Geometry: see drawing. Coordinates: mm, zero at the bounding-box minimum. A direction names the side the tool comes from. Round coordinates to 2 decimals unless told otherwise and drop trailing zeros. Loops run counter-clockwise (first coordinate to the right, second up) from the corner with the lowest first, then second, coordinate; pieces in that order, holes last. Notation, with made-up numbers: M 34,4 L 65,4 A30 ccw 65,39 Z; hole C 27.5,-32.75 d6. An arc over 180 degrees is marked long. Answer as a JSON object with one key per item and string values.
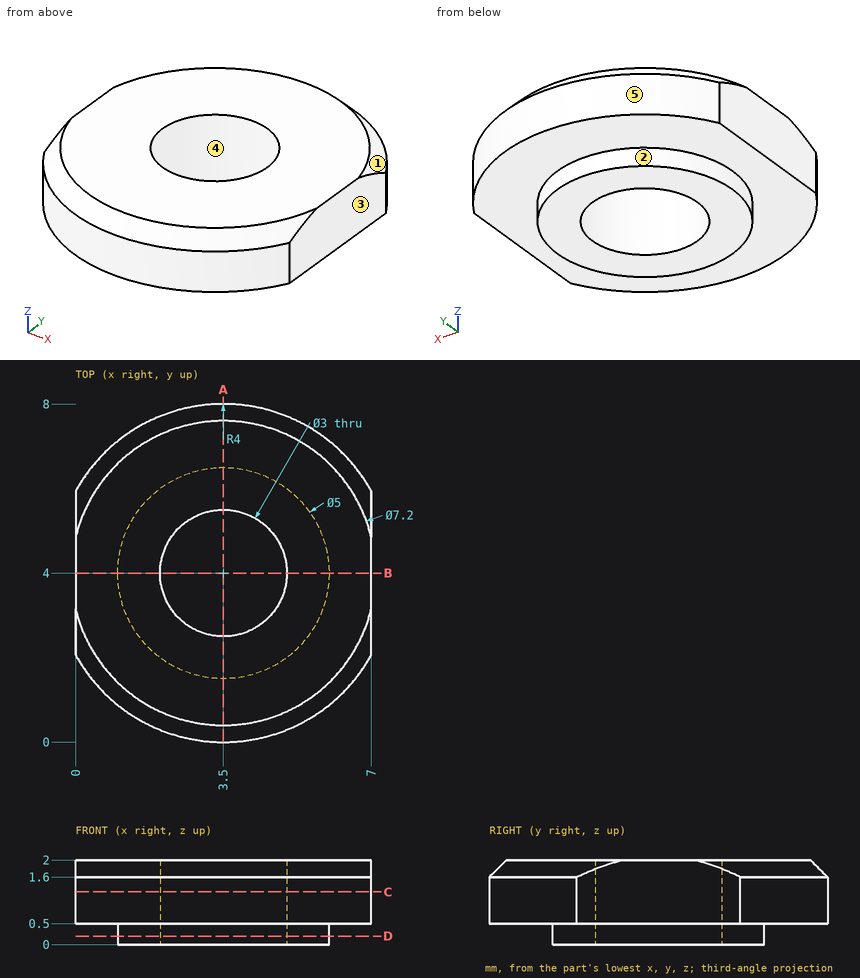
1) Section query B-B (y = 4). Return the cut outline in (x, z).
Results:
{"outline": "M 0,0.5 L 1,0.5 L 1,0 L 2,0 L 2,2 L 0,2 Z; M 5,0 L 6,0 L 6,0.5 L 7,0.5 L 7,2 L 5,2 Z"}
2) Section query C-C (z = 1.25). Return the cut outline in (x, y).
Results:
{"outline": "M 0,2.06 A4 ccw 7,2.06 L 7,5.94 A4 ccw 0,5.94 Z; hole C 3.5,4 d3"}
3) Pull-direction query (Y, two-part tool) for the marked faces 3, 4 and 5; classes: +Y half, -Y half, draft (parallel to the pull), parting line (faces both ways), or undercut.
Results:
{"face 3": "draft", "face 4": "undercut", "face 5": "+Y half"}
4) Reachability of the marked faces 1 and 2 from +Z, -Z, +X, -X, +Y, -Y: full face, straight path, thin tool, end or side. Return the list, or none.
Results:
{"face 1": "+Z, +Y", "face 2": "-Z"}
5) Pin query (flat end, axial travel): P1, Ø2.5, axis at x = 3.5, y = 4, coming from the +Z side. Return the tip coordinate at first contact, or that it passes through.
Results:
{"P1": "through"}
6) Ray query, line 1 (Z direction, x = 1, y = 4.75); line 2 (Y direction, x = 2.5, z = 1.2); line 3 (Y direction, x = 3.5, z = 0.4). Return the intervals inside material, ascending.
Results:
{"line 1": "0.5 to 2", "line 2": "0.13 to 2.88, 5.12 to 7.87", "line 3": "1.5 to 2.5, 5.5 to 6.5"}
7) Section query A-A (x = 3.5). Return the cut outline in (y, z).
Results:
{"outline": "M 0,0.5 L 1.5,0.5 L 1.5,0 L 2.5,0 L 2.5,2 L 0.4,2 L 0,1.6 Z; M 5.5,0 L 6.5,0 L 6.5,0.5 L 8,0.5 L 8,1.6 L 7.6,2 L 5.5,2 Z"}
8) Section query D-D (z = 0.2). Return the cut outline in (x, y), and give its area (3 significant figures).
Results:
{"outline": "C 3.5,4 d5; hole C 3.5,4 d3", "area": "12.6 mm2"}
